from build123d import *

# Parameters (mm, degrees)
F1_DEPTH = 20
F4_D     = 5.5
F3_R     = 5
F5_DEPTH = 15


with BuildPart() as f1:
    # F0 (on Right) → F1 (new body)
    with BuildSketch(Plane.YZ):
        Polygon((0, 20), (0, 0), (20, 0), align=None)
    extrude(amount=-F1_DEPTH)

    # F4 (through all)
    with Locations(Plane(origin=(0, 20, 0), x_dir=(1, 0, 0), z_dir=(0, 1, 0))):
        with Locations((-10, -10)):
            Hole(F4_D / 2)

    # F3 (on offset) → F5 (cut)
    with BuildSketch(Plane.XZ.offset(-20)):
        with Locations((-10, 10)):
            Circle(F3_R)
    extrude(amount=F5_DEPTH, mode=Mode.SUBTRACT)


solid = f1.part
Source: CAD feature listing. Evaluate the final solid. Frame: model axes, mm. A direction names the side the tool comes from. Round coordinates to 2 decimals unless told otherwise and drop trailing zeros. Loops run counter-clockwise (first coordinate to the right, second up) from the corner with the lowest first, then second, coordinate; pieces in that order, holes last. Notation, with made-up numbers: (-16, -1) -> (15, -1) arc R28 cw to (15, 35) -> close; hole circle Ø1 at (-27.75, 60.25). An arc over 180 degrees is marked (long way). Answer as a JSON object with one key per item and string values. Group by question number.
Q1. Section query D-D (y = 9). Output: boundary loops of the cut face in (x, z), plus the area to 3 significant figures.
Q2. Section query B-B (x = -6). Output: boundary loops of the cut face in (y, z), plus the area to 3 significant figures.
Q3. Section query A-A (z = 10). Output: boundary loops of the cut face in (x, y).
Q4. Ray query, line 1 (X direction, y = 2.1, z = 10); line 2 (Z direction, x = -10, y = 10.5). Return the intervals inside material, ascending. Write a range as from..to.
Q5. Contact query for flat-ended pins moving along their axis: P1, Ø12, axis at x = -14, y = 8, coming from the +Z side; P2, Ø2, axis at x = -9.5, z = 4, coming from the -Y side; P3, Ø9, axis at x = -10, z = 10, coming from the +Y side; P4, Ø11, axis at x = -8, z = 8.5, coming from the +Y side. Output: stop coordinate, or through.
Q6. Mould query, pull axis X, two halves, no side actions, for faces 1 (the flat face through (-7.8, 5, 7.8)), 2 (the flat face through (0, 5, 6)), 3 (the flat face through (-10, 10, 0)). Classes: pulls with the +X half, pulls with the -X half, needs draft (parallel to the pull), parting line crosses it, or undercut.
Q7. Access query for faces 4 (the cylindrical face through (-11.08, 8.96, 5.12)), 5 (the cylindrical face through (-12.62, 2.46, 9.17)). Directions: +Z, -Z, +X, -X, +Y, -Y. A direction counts if a zero-diameter tool reaches every point of the face in a straight line with its end or side. Return the directions, or none.
Q8. Section query C-C (x = -8). Output: boundary loops of the cut face in (y, z).
Completed:
{
 "1": {"outline": "(-20, 0) -> (0, 0) -> (0, 11) -> (-5.1, 11) arc R5 cw (long way) to (-14.9, 11) -> (-20, 11) -> close", "area": "171 mm²"},
 "2": {"outline": "(0, 0) -> (20, 0) -> (13, 7) -> (5, 7) -> (5, 13) -> (7, 13) -> (0, 20) -> close", "area": "170 mm²"},
 "3": {"outline": "(-20, 0) -> (-12.75, 0) -> (-12.75, 5) -> (-15, 5) -> (-15, 10) -> (-20, 10) -> close; (-7.25, 0) -> (0, 0) -> (0, 10) -> (-5, 10) -> (-5, 5) -> (-7.25, 5) -> close"},
 "4": {"line 1": "-20..-12.75, -7.25..0", "line 2": "0..5"},
 "5": {"P1": "z = 18", "P2": "y = 0", "P3": "y = 5", "P4": "y = 17"},
 "6": {"face 1": "undercut", "face 2": "pulls with the +X half", "face 3": "needs draft"},
 "7": {"face 4": "+Y", "face 5": "+Y, -Y"},
 "8": {"outline": "(0, 0) -> (20, 0) -> (14.58, 5.42) -> (5, 5.42) -> (5, 8.11) -> (0, 8.11) -> close; (0, 11.89) -> (5, 11.89) -> (5, 14.58) -> (5.42, 14.58) -> (0, 20) -> close"}
}
